Autodesk Inventor part; units mm, degrees
ref_plane "Work Plane1" through (0, 0, 80) normal (0, 0, 1) x (1, 0, 0)
ref_plane "YZ Plane" through (0, 0, 0) normal (1, 0, 0) x (0, 1, 0)
ref_plane "XZ Plane" through (0, 0, 0) normal (0, 1, 0) x (-1, 0, 0)
sketch "Sketch4" plane through (0, 0, 0) normal (0, 0, 1) x (1, 0, 0)
  line L0 (-27.5, 17.5) -> (27.5, 17.5)
  line L1 (27.5, 17.5) -> (27.5, -17.5)
  line L2 (27.5, -17.5) -> (-27.5, -17.5)
  line L3 (-27.5, -17.5) -> (-27.5, 17.5)
  line L4 (0, 0) -> (0, -2.5)
  line L5 (0, 0) -> (1.7044, 0)
  dimension "d52" = 55
  dimension "d53" = 35
extrude "Extrusion3" add sketch "Sketch4" along normal blind 15
sketch "Sketch1" plane through (0, 0, 0) normal (0, 0, -1) x (-1, 0, 0)
  line L0 (-25.5, 15.5) -> (25.5, 15.5)
  line L1 (25.5, 15.5) -> (25.5, -15.5)
  line L2 (25.5, -15.5) -> (-25.5, -15.5)
  line L3 (-25.5, -15.5) -> (-25.5, 15.5)
  line L4 (27.5, 17.5) -> (-27.5, 17.5)
  line L5 (-27.5, 17.5) -> (-27.5, -17.5)
  line L6 (-27.5, -17.5) -> (27.5, -17.5)
  line L7 (27.5, -17.5) -> (27.5, 17.5)
  line L8 (0, 0) -> (0, -2)
  line L9 (0, 0) -> (2, 0)
  dimension "d0" = 51
  dimension "d1" = 31
extrude "Extrusion4" cut sketch "Sketch1" against normal blind 10 contours L0 L1 L2 L3
sketch "Sketch5" plane through (0, 0, 10) normal (0, 0, -1) x (-1, 0, 0)
  line L0 (-25.5, 15.5) -> (25.5, 15.5)
  line L1 (-25.5, -15.5) -> (-25.5, 15.5)
  line L2 (25.5, -15.5) -> (-25.5, -15.5)
  line L3 (25.5, 15.5) -> (25.5, -15.5)
  line L4 (0, 0) -> (2, 0)
  line L5 (0, 0) -> (0, -2)
  line L6 (-20.5, 10.5) -> (20.5, 10.5)
  line L7 (20.5, 10.5) -> (20.5, -10.5)
  line L8 (20.5, -10.5) -> (-20.5, -10.5)
  line L9 (-20.5, -10.5) -> (-20.5, 10.5)
  dimension "d58" = 2
  dimension "d59" = 2
  dimension "d60" = 41
  dimension "d61" = 21
extrude "Extrusion5" cut sketch "Sketch5" against normal blind 5 contours L6 L7 L8 L9
sketch "Sketch2" plane through (0, 0, 80) normal (0, 0, 1) x (1, 0, 0)
  circle A0 centre (0, 0) radius 55
  dimension "d6" = 110
sketch "Sketch3" plane through (0, 0, 80) normal (0, 0, 1) x (1, 0, 0)
  circle A0 centre (0, 0) radius 52
  dimension "d30" = 104
properties part number "embudo0.2"
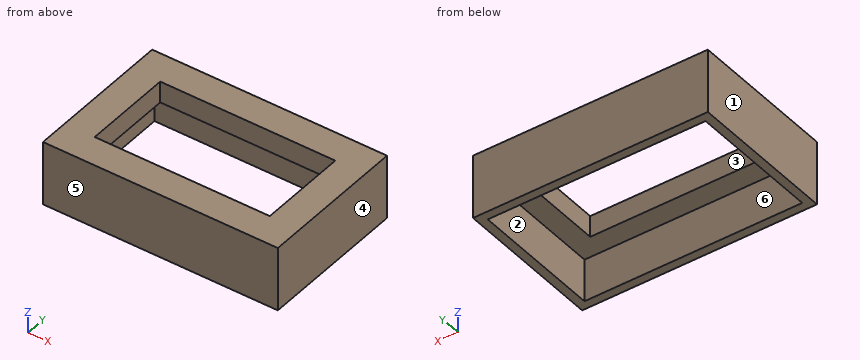
Source: CAD feature listing. Evaluate the final solid. Frame: model axes, mm. Face numbers are marked on the shaded views. A direction names the side the tool comes from. Give positions to 0.01 mm unless a question says otherwise; leave off trailing zeros. Loops run counter-clockwise (first coordinate to the right, second up) from the corner with the lowest first, then second, coordinate; pieces in that order, holes last. Notation, with made-up numbers: (67.25, 24) -> (84.25, 24) arc R7 ccw to (84.25, 34) -> close; hole circle Ø4 at (49.25, -1.5). An arc over 180 degrees is marked (long way). Put each result on its own line as item: value. Start each with the question number.
1) Material intervals for probe 1 along X at (y, z) = (-6.5, 13); probe 2 along Y at (x, z) = (13, 5.25); probe 3 along X at (y, z) = (10, 2.75), sorted ascending.
2) Reachability of the marked faces 1, 2 and 3 from +Z, -Z, +X, -X, +Y, -Y: full face, straight path, thin tool, end or side. Return the list, or none.
3) Cut plane B-B (y = 9). Return loops of the section in (x, z), then the cut area to 3 significant figures.
4) Cut plane A-A (z = 2). Return loops of the section in (x, y).
5) Draft query along X for the marked faces 4, 5 and 6. Return one class per face: released by +X, released by -X, zero draft, split by the parting line, or undercut.
6) Cut plane C-C (x = -18.5). Return loops of the section in (y, z).
7) Contact query for flat-ended pins moving along their axis: P1, Ø10, axis at x = -13, y = 6, coming from the -Z side; P2, Ø9.5, axis at x = -11.5, y = 4, coming from the -Z side. Output: stop coordinate, or through.
8) Cut plane D-D (y = 12.5). Return loops of the section in (x, z), then the cut area to 3 significant figures.
Results are:
1. probe 1: x = -27.5 to -20.5, 20.5 to 27.5
1. probe 2: y = -17.5 to -15.5, 15.5 to 17.5
1. probe 3: x = -27.5 to -25.5, 25.5 to 27.5
2. face 1: +Z, -Z, -X, +Y, -Y
2. face 2: -Z
2. face 3: +Z, -Z
3. outline: (-27.5, 0) -> (-25.5, 0) -> (-25.5, 10) -> (-20.5, 10) -> (-20.5, 15) -> (-27.5, 15) -> close; (20.5, 10) -> (25.5, 10) -> (25.5, 0) -> (27.5, 0) -> (27.5, 15) -> (20.5, 15) -> close
3. area: 110 mm2
4. outline: (-27.5, -17.5) -> (27.5, -17.5) -> (27.5, 17.5) -> (-27.5, 17.5) -> close; hole (-25.5, -15.5) -> (25.5, -15.5) -> (25.5, 15.5) -> (-25.5, 15.5) -> close
5. face 4: released by +X
5. face 5: zero draft
5. face 6: undercut
6. outline: (-17.5, 0) -> (-15.5, 0) -> (-15.5, 10) -> (-10.5, 10) -> (-10.5, 15) -> (-17.5, 15) -> close; (10.5, 10) -> (15.5, 10) -> (15.5, 0) -> (17.5, 0) -> (17.5, 15) -> (10.5, 15) -> close
7. P1: stops at z = 10
7. P2: passes through
8. outline: (-27.5, 0) -> (-25.5, 0) -> (-25.5, 10) -> (25.5, 10) -> (25.5, 0) -> (27.5, 0) -> (27.5, 15) -> (-27.5, 15) -> close
8. area: 315 mm2
